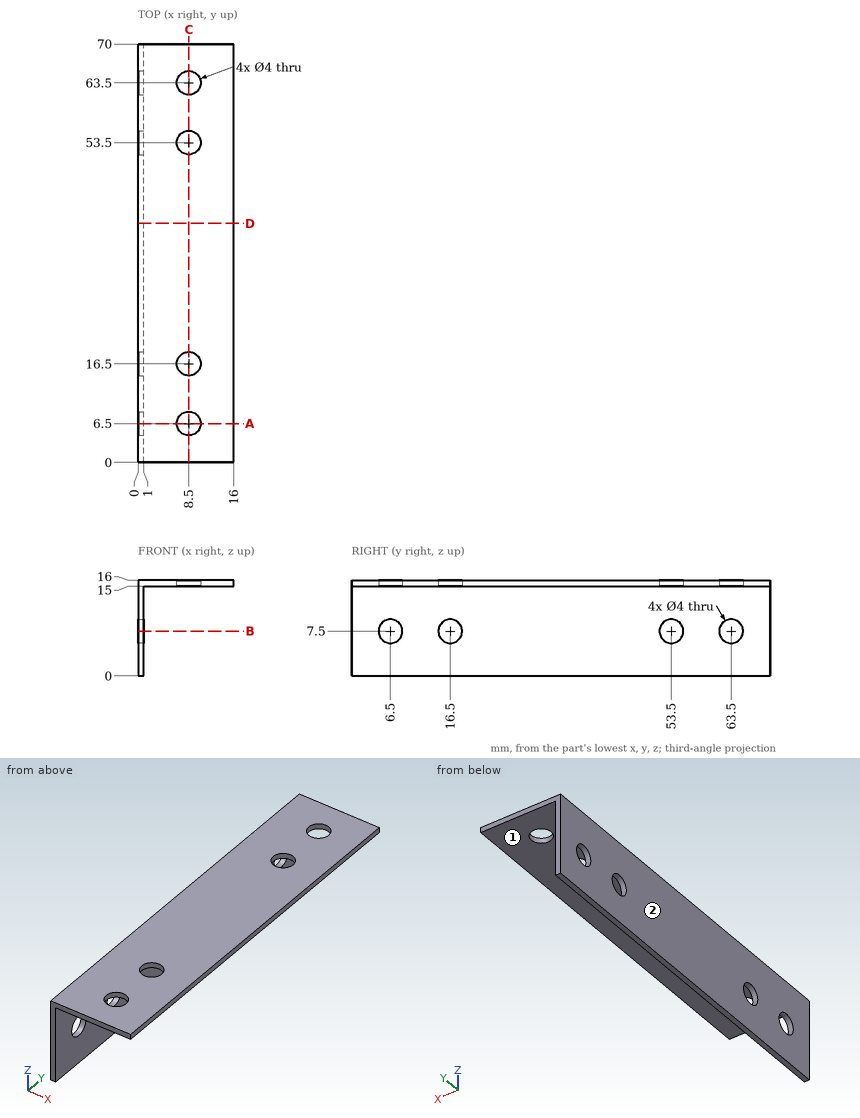
Input: dimensioned drawing with shaded views. Units: mm. Origin: part minimum x, y, z. A direction names the side the tool comes from. Coordinates: 2 decimals unless noted, no trailing zeros. Loops run counter-clockwise (first coordinate to the right, second up) from the corner with the lowest first, then second, coordinate; pieces in that order, holes last. Notation, with made-up numbers: M -5,48.5 L 26,48.5 A9 ccw 26,65.5 Z; hole C -21,-24.5 d3. An arc over 180 degrees is marked long. One line per item, written item: value. Start each with the question number.
1) Cut plane A-A (y = 6.5). Return loops of the section in (x, z).
2) Cut plane B-B (z = 7.5). Return loops of the section in (x, y), then the cut area to 3 significant figures.
3) Reachability of the marked faces 1 and 2 from +Z, -Z, +X, -X, +Y, -Y: full face, straight path, thin tool, end or side. Return the list, or none.
4) Cut plane C-C (x = 8.5). Return loops of the section in (y, z).
5) Material intervals for L1, parallel to Y at x = 8.5, z = 15.45; L2, parallel to X at y = 9, z = 11.5; L3, parallel to Z at x = 3.5, y = 15.5, sorted ascending. Write a range as from..to.
6) Pin query (flat end, axial travel): P1, Ø5, axis at y = 6.5, z = 7.5, coming from the -X side; P2, Ø4, axis at x = 5.5, y = 35, coming from the -Z side. Return the tip coordinate at first contact, or that it passes through.
7) Cut plane D-D (y = 40). Return loops of the section in (x, z), then the cut area to 3 significant figures.
Evaluation:
1. outline: M 0,0 L 1,0 L 1,5.5 L 0,5.5 Z; M 0,9.5 L 1,9.5 L 1,15 L 6.5,15 L 6.5,16 L 0,16 Z; M 10.5,15 L 16,15 L 16,16 L 10.5,16 Z
2. outline: M 0,0 L 1,0 L 1,4.5 L 0,4.5 Z; M 0,8.5 L 1,8.5 L 1,14.5 L 0,14.5 Z; M 0,18.5 L 1,18.5 L 1,51.5 L 0,51.5 Z; M 0,55.5 L 1,55.5 L 1,61.5 L 0,61.5 Z; M 0,65.5 L 1,65.5 L 1,70 L 0,70 Z
2. area: 54.0 mm^2
3. face 1: -Z, +X, +Y, -Y
3. face 2: +Z, -Z, -X, +Y, -Y
4. outline: M 0,15 L 4.5,15 L 4.5,16 L 0,16 Z; M 8.5,15 L 14.5,15 L 14.5,16 L 8.5,16 Z; M 18.5,15 L 51.5,15 L 51.5,16 L 18.5,16 Z; M 55.5,15 L 61.5,15 L 61.5,16 L 55.5,16 Z; M 65.5,15 L 70,15 L 70,16 L 65.5,16 Z
5. L1: 0..4.5, 8.5..14.5, 18.5..51.5, 55.5..61.5, 65.5..70
5. L2: 0..1
5. L3: 15..16
6. P1: x = 0
6. P2: z = 15
7. outline: M 0,0 L 1,0 L 1,15 L 16,15 L 16,16 L 0,16 Z
7. area: 31.0 mm^2
